Geometry check sheet. Reference: the model listing, model coordinates, mm. A direction names the side the tool comes from. Round coordinates to 2 decimals unless told otherwise and drop trailing zeros. Write each loop counter-clockwise with the first axis right and the second up, starting at its lowest first coordinate (ties: lowest second). Pieces come first, ordered by that corner, then holes. Notation, with made-up numbers: M 41,87 L 80,87 A24 ccw 80,120 Z; hole C 78.5,18 d2. An arc over 180 degrees is marked long. One line per item, written item: value. Start each with the question number.
1. Section check B-B (y = -3.25). Record the boundary of the cut face in (x, z), and give its area (4 significant figures).
2. Scan lines: probe 1 along Y at (x, z) = (103.5, 2.25); probe 2 along Z at (x, y) = (30, -2.75); probe 3 along Z at (x, y) = (-10, 4.25). Record each from-to range of solid material in increasing order. Write a range as [from, to].
3. Section check A-A (x = 101). Record the boundary of the cut face in (y, z), and give its area (3 significant figures).
4. Depth check by flat-ended pin: P1, Ø4, axis at x = 18.5, y = 0.5, coming from the +Z side; P2, Ø5, axis at x = 7, y = -0.5, coming from the -Z side; P3, Ø1.5, axis at x = 41.5, z = 3.5, coming from the -Y side. Enter the tip coordinate at first touch or a pass-through.
5. Access from +Z, -Z, +X, -X, +Y, -Y to the whole of each face (thin tool, end or side, straight path). Record for faces 1 (the flat face through (-2, 4, 6)), 2 (the flat face through (-2, 5, 6)).
Autodesk Inventor part; units mm, degrees
ref_plane "YZ Plane" through (0, 0, 0) normal (1, 0, 0) x (0, 1, 0)
ref_plane "XZ Plane" through (0, 0, 0) normal (0, 1, 0) x (-1, 0, 0)
ref_plane "XY Plane" through (0, 0, 0) normal (0, 0, 1) x (1, 0, 0)
sketch "Sketch1" plane through (0, 0, 0) normal (0, 0, 1) x (1, 0, 0)
  line L0 (-125, -5) -> (125, -5)
  line L1 (125, -5) -> (125, 5)
  line L2 (125, 5) -> (-125, 5)
  line L3 (-125, 5) -> (-125, -5)
  line L4 (-125, -5) -> (125, 5) construction
  line L5 (125, -5) -> (-125, 5) construction
  point P0 (0, 0)
  dimension "d0" = 250
  dimension "d1" = 10
extrude "Plate1" add sketch "Sketch1" along normal blind 1
sketch "Sketch2" plane through (-125, 4, 0) normal (0, 1, 0) x (-1, 0, 0)
  line L0 (-250, 0) -> (0, 0)
  line L1 (0, 0) -> (0, 10)
  line L2 (0, 10) -> (-250, 10)
  line L3 (-250, 10) -> (-250, 0)
edge flange "Flange1" height 10 angle 90 thickness 1 bend radius 1 thickness toward (0, 1, 0) relief tear relief width 1 relief depth 0.5 edges at (0, 5, 1) wall of the first edge with corners at (125, 4, 0) (-125, 4, 0) (-125, 4, 10) (125, 4, 10)
bend "Bend1"
corner "Corner1"
chamfer "Corner Chamfer1" distance 4 angle 45 4 edges at (-125, 4.5, 10) (125, -5, 0.5) (125, 4.5, 10) (-125, -5, 0.5)
equation "\"d3\" = BendReliefWidth"
equation "\"d4\" = BendReliefDepth"
equation "\"d5\" = MinimumRemnant"
equation "\"d6\" = BendRadius"
equation "\"d9\" = BendRadius"
equation "\"d10\" = CornerReliefSize"
equation "\"d11\" = GapSize"
equation "\"d12\" = JacobiRadiusSize"
equation "\"BendRadius\" = Thickness"
equation "\"BendReliefWidth\" = Thickness"
equation "\"BendReliefDepth\" = 0.5 * Thickness"
equation "\"CornerReliefSize\" = 4 * Thickness"
equation "\"MinimumRemnant\" = 2 * Thickness"
equation "\"TransitionRadius\" = BendRadius"
equation "\"JacobiRadiusSize\" = BendRadius"
equation "\"GapSize\" = Thickness"
equation "\"d2\" = BendRadius"
Result sheet:
1. outline: M -122.75,0 L 122.75,0 L 122.75,1 L -122.75,1 Z
1. area: 245.5 mm2
2. probe 1: y = [4, 5]
2. probe 2: z = [0, 1]
2. probe 3: z = [0.44, 10]
3. outline: M -5,0 L 3,0 A2 ccw 5,2 L 5,10 L 4,10 L 4,2 A1 cw 3,1 L -5,1 Z
3. area: 18.4 mm2
4. P1: stops at z = 1
4. P2: stops at z = 0
4. P3: stops at y = 4
5. face 1: +Z, +X, -X, -Y
5. face 2: +Z, -Z, +X, -X, +Y
